from build123d import *

# Parameters (mm, degrees)
BOSS_EXTRUDE2_DEPTH = 3.175
SKETCH3_R           = 3.571875
BOSS_EXTRUDE3_DEPTH = 3.175
CUT_EXTRUDE1_REACH  = 8.35
SKETCH4_R           = 1.5875
FILLET1_R           = 3.175
FILLET2_R           = 0.79375
CHAMFER1_SIZE       = 0.508
CHAMFER2_SIZE       = 0.254


with BuildPart() as part:
    # Sketch2 → Boss-Extrude2 (new body)
    with BuildSketch(Plane(origin=(0, 0, 0), x_dir=(1, 0, 0), z_dir=(0, 1, 0))):
        Polygon((-39.0525, -13.97), (-39.0525, -3.175), (39.0525, -3.175), (39.0525, -13.97), (49.8475, -13.97), (49.8475, -3.175), (52.71135, 3.175), (52.71135, 13.3477), (42.53865, 13.3477), (42.53865, 3.175), (-42.53865, 3.175), (-42.53865, 13.3477), (-52.71135, 13.3477), (-52.71135, 3.175), (-49.8475, -3.175), (-49.8475, -13.97), align=None)
    extrude(amount=BOSS_EXTRUDE2_DEPTH)

    # Sketch3 → Boss-Extrude3 (add)
    with BuildSketch(Plane(origin=(0, 3.175, 0), x_dir=(1, 0, 0), z_dir=(0, 1, 0))):
        with Locations((-47.625, 8.26135)):
            Circle(SKETCH3_R)
        with Locations((-44.45, -8.5725)):
            Circle(SKETCH3_R)
        with Locations((44.45, -8.5725)):
            Circle(SKETCH3_R)
        with Locations((47.625, 8.26135)):
            Circle(SKETCH3_R)
    extrude(amount=BOSS_EXTRUDE3_DEPTH)

    # Sketch4 → Cut-Extrude1 (cut, up to next)
    with BuildSketch(Plane.XZ, mode=Mode.PRIVATE) as cut_extrude1_sk1:
        with Locations((-44.45, 8.5725)):
            Circle(SKETCH4_R)
    cut_extrude1_tool1 = extrude(cut_extrude1_sk1.sketch, amount=-CUT_EXTRUDE1_REACH, mode=Mode.PRIVATE) & part.part
    add(cut_extrude1_tool1.solids().sort_by_distance((-44.45, 0, 8.5725))[0], mode=Mode.SUBTRACT)
    # Sketch4 → Cut-Extrude1 (cut, up to next)
    with BuildSketch(Plane.XZ, mode=Mode.PRIVATE) as cut_extrude1_sk2:
        with Locations((-47.625, -8.26135)):
            Circle(SKETCH4_R)
    cut_extrude1_tool2 = extrude(cut_extrude1_sk2.sketch, amount=-CUT_EXTRUDE1_REACH, mode=Mode.PRIVATE) & part.part
    add(cut_extrude1_tool2.solids().sort_by_distance((-47.625, 0, -8.26135))[0], mode=Mode.SUBTRACT)
    # Sketch4 → Cut-Extrude1 (cut, up to next)
    with BuildSketch(Plane.XZ, mode=Mode.PRIVATE) as cut_extrude1_sk3:
        with Locations((47.625, -8.26135)):
            Circle(SKETCH4_R)
    cut_extrude1_tool3 = extrude(cut_extrude1_sk3.sketch, amount=-CUT_EXTRUDE1_REACH, mode=Mode.PRIVATE) & part.part
    add(cut_extrude1_tool3.solids().sort_by_distance((47.625, 0, -8.26135))[0], mode=Mode.SUBTRACT)
    # Sketch4 → Cut-Extrude1 (cut, up to next)
    with BuildSketch(Plane.XZ, mode=Mode.PRIVATE) as cut_extrude1_sk4:
        with Locations((44.45, 8.5725)):
            Circle(SKETCH4_R)
    cut_extrude1_tool4 = extrude(cut_extrude1_sk4.sketch, amount=-CUT_EXTRUDE1_REACH, mode=Mode.PRIVATE) & part.part
    add(cut_extrude1_tool4.solids().sort_by_distance((44.45, 0, 8.5725))[0], mode=Mode.SUBTRACT)

    # Fillet1
    fillet1_edges = [part.edges().sort_by_distance(p)[0] for p in [
        (-42.53865, 1.5875, -13.3477),
        (-42.53865, 1.5875, -3.175),
        (42.53865, 1.5875, -3.175),
        (42.53865, 1.5875, -13.3477),
        (52.71135, 1.5875, -13.3477),
        (52.71135, 1.5875, -3.175),
        (49.8475, 1.5875, 3.175),
        (49.8475, 1.5875, 13.97),
        (39.0525, 1.5875, 13.97),
        (39.0525, 1.5875, 3.175),
        (-39.0525, 1.5875, 3.175),
        (-39.0525, 1.5875, 13.97),
        (-49.8475, 1.5875, 13.97),
        (-49.8475, 1.5875, 3.175),
        (-52.71135, 1.5875, -3.175),
        (-52.71135, 1.5875, -13.3477),
    ]]
    fillet(fillet1_edges, radius=FILLET1_R)

    # Fillet2
    fillet2_edges = [part.edges().sort_by_distance(p)[0] for p in [
        (-51.196875, 3.175, -8.26135),
        (-48.021875, 3.175, 8.5725),
        (44.053125, 3.175, -8.26135),
        (40.878125, 3.175, 8.5725),
    ]]
    fillet(fillet2_edges, radius=FILLET2_R)

    # Chamfer1
    chamfer1_edges = [part.edges().sort_by_distance(p)[0] for p in [
        (51.78141403, 0, -12.41776403),
        (43.46858597, 0, -12.41776403),
        (-43.46858597, 0, -12.41776403),
        (-42.53865, 3.175, -8.26135),
        (-52.71135, 3.175, -7.015272864),
        (-51.279425, 3.175, 0),
        (-49.8475, 3.175, 7.326422864),
        (-44.45, 3.175, 13.97),
        (-39.0525, 3.175, 8.5725),
        (0, 3.175, 3.175),
        (39.0525, 3.175, 8.5725),
        (44.45, 3.175, 13.97),
        (49.8475, 3.175, 7.326422864),
        (51.279425, 3.175, 0),
        (52.71135, 3.175, -7.015272864),
        (47.625, 3.175, -13.3477),
        (42.53865, 3.175, -8.26135),
        (0, 3.175, -3.175),
        (-51.78141403, 3.175, -12.41776403),
        (-52.640373335, 3.175, -3.190264917),
        (-48.91756403, 3.175, 13.04006403),
        (-39.98243597, 3.175, 13.04006403),
        (39.98243597, 3.175, 13.04006403),
        (48.91756403, 3.175, 13.04006403),
        (52.640373335, 3.175, -3.190264917),
        (51.78141403, 3.175, -12.41776403),
        (43.46858597, 3.175, -12.41776403),
        (-43.46858597, 3.175, -12.41776403),
        (-41.60871403, 0, -4.10493597),
        (-41.60871403, 3.175, -4.10493597),
        (41.60871403, 0, -4.10493597),
        (41.60871403, 3.175, -4.10493597),
        (49.918476665, 0, 3.190264917),
        (49.918476665, 3.175, 3.190264917),
        (38.12256403, 0, 4.10493597),
        (38.12256403, 3.175, 4.10493597),
        (-49.918476665, 0, 3.190264917),
        (-49.918476665, 3.175, 3.190264917),
        (-38.12256403, 0, 4.10493597),
        (-38.12256403, 3.175, 4.10493597),
        (-47.625, 0, -13.3477),
        (-47.625, 3.175, -13.3477),
        (-42.53865, 0, -8.26135),
        (0, 0, -3.175),
        (42.53865, 0, -8.26135),
        (47.625, 0, -13.3477),
        (52.71135, 0, -7.015272864),
        (51.279425, 0, 0),
        (49.8475, 0, 7.326422864),
        (44.45, 0, 13.97),
        (39.0525, 0, 8.5725),
        (0, 0, 3.175),
        (-39.0525, 0, 8.5725),
        (-44.45, 0, 13.97),
        (-49.8475, 0, 7.326422864),
        (-51.279425, 0, 0),
        (-52.71135, 0, -7.015272864),
        (-51.78141403, 0, -12.41776403),
        (-52.640373335, 0, -3.190264917),
        (-48.91756403, 0, 13.04006403),
        (-39.98243597, 0, 13.04006403),
        (39.98243597, 0, 13.04006403),
        (48.91756403, 0, 13.04006403),
        (52.640373335, 0, -3.190264917),
    ]]
    chamfer(chamfer1_edges, length=CHAMFER1_SIZE)

    # Chamfer2
    chamfer2_edges = [part.edges().sort_by_distance(p)[0] for p in [
        (-51.196875, 6.35, -8.26135),
        (-48.021875, 6.35, 8.5725),
        (44.053125, 6.35, -8.26135),
        (40.878125, 6.35, 8.5725),
        (42.8625, 6.35, 8.5725),
        (42.8625, 0, 8.5725),
        (46.0375, 6.35, -8.26135),
        (46.0375, 0, -8.26135),
        (-49.2125, 6.35, -8.26135),
        (-49.2125, 0, -8.26135),
        (-46.0375, 6.35, 8.5725),
        (-46.0375, 0, 8.5725),
    ]]
    chamfer(chamfer2_edges, length=CHAMFER2_SIZE)


solid = part.part
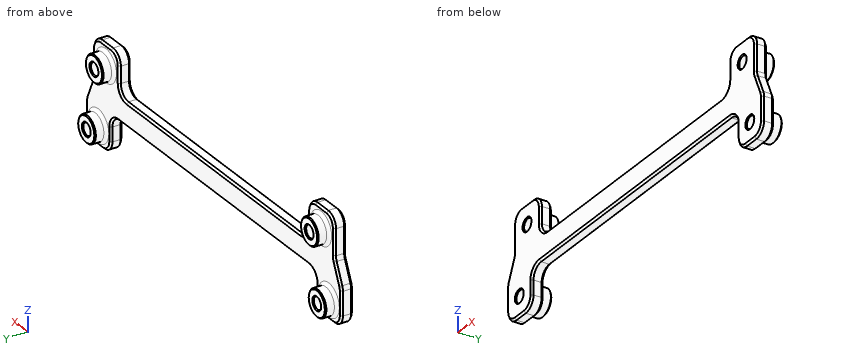
Geometry: final body of the model. Coordinates: model frame, mm. Give positions to 0.01 mm unless a question says otherwise; leave off trailing zeros. Write each loop counter-clockwise with the first axis right and the second up, starting at its lowest first coordinate (ties: lowest second). Pieces come first, ordered by that corner, then holes. Notation, with made-up numbers: M 88.25,-10.75 L 132.25,-10.75 A9 ccw 132.25,-3.75 Z; hole C 65,-7 d3. An arc over 180 degrees is marked long. Answer in a Markdown table with one row per item. Add a question column.
(1) Section A-A on x = -12. Return loops of the section in (y, z) (3 decimals).
(2) Ray query, line 1 (X direction, y = 1.5, z = -8); line 2 (Z direction, x = -44.45, y = 4.9) (3 decimals); line 3 (X direction, y = 5.75, z = 8.25). Return the intervals inside material, ascending.
(3) Section B-B on y = 1.75. State how many separate pieces and enclosed holes the cut face has, and give its area (3 significant figures).
(4) First-contact query: pin 1 (3.5 mm diameter, centred on x = 47.62, z = -8.26, fed in from -Y); pin 2 (1.1 mm diameter, centred on x = 5, y = 1, fed in from +Z) (3 decimals); pin 3 (1.7 mm diameter, centred on x = -14.5, y = 1.5, fed in from -Z) (3 decimals). Flat tips, straight axial feed; report the tip coordinate or a pass-through.
Result set:
| question | item | result |
|---|---|---|
| 1 | outline | M 0,-2.667 L 0.508,-3.175 L 2.667,-3.175 L 3.175,-2.667 L 3.175,2.667 L 2.667,3.175 L 0.508,3.175 L 0,2.667 Z |
| 2 | line 1 | x = -52.71 to -49.19, -46.06 to -42.54, 42.54 to 46.06, 49.19 to 52.71 |
| 2 | line 2 | z = -9.898 to -6.625, 5.001 to 6.985, 10.16 to 12.144 |
| 2 | line 3 | x = -48.01 to -46, -42.9 to -40.89, 40.89 to 42.9, 46 to 48.01 |
| 3 | separate pieces | 1 |
| 3 | enclosed holes | 4 |
| 3 | area | 1,050 mm^2 |
| 4 | pin 1 | stops at y = 0.09 |
| 4 | pin 2 | stops at z = 3.175 |
| 4 | pin 3 | stops at z = -3.175 |
